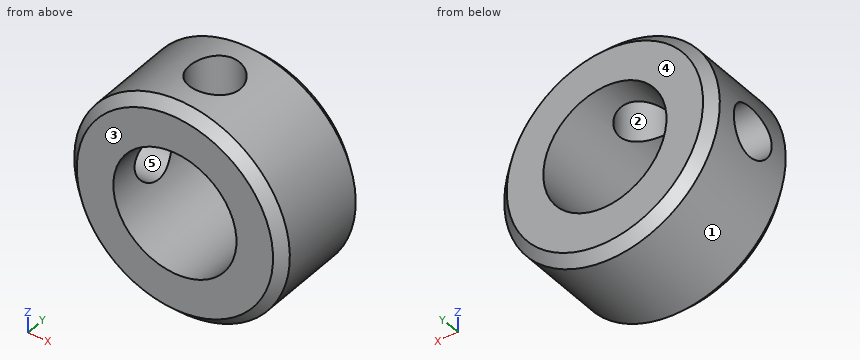
from build123d import *

# Parameters (mm, degrees)
SKETCH1_R                  = 7
SKETCH1_R_2                = 4
BOSS_EXTRUDE1_DEPTH        = 3.5
M4X0_7_TAPPED_HOLE1_REACH  = 18.039
M4X0_7_TAPPED_HOLE1_BORE_R = 1.65
CHAMFER1_SIZE              = 0.625
CIRPATTERN1_COUNT          = 2
CIRPATTERN1_ANGLE          = 90


with BuildPart() as part:
    # Sketch1 → Boss-Extrude1 (new, symmetric)
    with BuildSketch(Plane(origin=(0, 0, 0), x_dir=(1, 0, 0), z_dir=(0, 1, 0))):
        with Locations(Location((0, 0, 0), (0, 0, 270))):
            Circle(SKETCH1_R)
        with Locations(Location((0, 0, 0), (0, 0, 270))):
            Circle(SKETCH1_R_2, mode=Mode.SUBTRACT)
    extrude(amount=BOSS_EXTRUDE1_DEPTH, both=True)

    # M4x0.7 Tapped Hole1 bore → M4x0.7 Tapped Hole1 (cut, up to next)
    with BuildSketch(Plane.XY.offset(7), mode=Mode.PRIVATE) as m4x0_7_tapped_hole1_sk1:
        Circle(M4X0_7_TAPPED_HOLE1_BORE_R)
    m4x0_7_tapped_hole1_tool1 = extrude(m4x0_7_tapped_hole1_sk1.sketch, amount=-M4X0_7_TAPPED_HOLE1_REACH, mode=Mode.PRIVATE) & part.part
    m4x0_7_tapped_hole1 = m4x0_7_tapped_hole1_tool1.solids().sort_by_distance((0, 0, 7))[0]
    add(m4x0_7_tapped_hole1, mode=Mode.SUBTRACT)

    # Chamfer1
    chamfer1_edges = [part.edges().sort_by_distance(p)[0] for p in [
        (0, -3.5, -7),
        (0, 3.5, -7),
    ]]
    chamfer(chamfer1_edges, length=CHAMFER1_SIZE)

    # CirPattern1: M4x0.7 Tapped Hole1 ×2 about axis
    cirpattern1_axis = Axis((0, 3.5, 0), (0, -1, 0))
    for i in range(1, CIRPATTERN1_COUNT):
        add(m4x0_7_tapped_hole1.rotate(cirpattern1_axis, i * CIRPATTERN1_ANGLE / (CIRPATTERN1_COUNT - 1)), mode=Mode.SUBTRACT)


solid = part.part
Build history of the part. All positions in model axes, mm. Face numbers are marked on the shaded views. A direction names the side the tool comes from. Round coordinates to 2 decimals unless told otherwise and drop trailing zeros. Write each loop counter-clockwise with the first axis right and the second up, starting at its lowest first coordinate (ties: lowest second). Pieces come first, ordered by that corner, then holes. Notation, with made-up numbers: M 83.5,0.25 L 108.5,0.25 A26 cw 108.5,26.25 Z; hole C 43,-26 d5. An arc over 180 degrees is marked long. Answer as a JSON object with one key per item and string values. Group by question number.
(1) Cut at B-B (x = 0). Give the cut face in (y, z) (3 decimals).
(2) Which spindle directions (+Z, -Z, +X, -X, +Y, -Y) get a long thin tool onto all of the face, cutting with end or side? Do the marked faces 1 and 2. Say none if no direction does.
(3) Cut at A-A (z = 0). Give the cut face in (x, y) (3 decimals).
(4) Drill centre lines: L1, parallel to Y at x = 0, z = 5.75; L2, parallel to X at y = 1, z = 1.5; L3, parallel to X at y = 2, z = 3. Where is each one in solid material? Low to high.
(5) Flat gauge pins, fed straight in: pin 1 (4 mm diameter, centred on x = 3, y = -2, fed in from -Z); pin 2 (1.5 mm diameter, centred on x = -5, y = 3, fed in from -Z); pin 3 (2 mm diameter, centred on x = 0, y = 0, fed in from +Z). Where does each tip first touch, or does it go through?
(6) Mould opens along Y. For the marked faces 3, 4 and 5 say: pulls with the +Y half, pulls with the -Y half, needs draft (parallel to the pull), parting line crosses it, or undercut.
(7) Cut at C-C (y = -2.25). Give the cut face in (x, z).
Responses:
{
 "1": {"outline": "M -3.5,-6.375 L -2.875,-7 L 2.875,-7 L 3.5,-6.375 L 3.5,-4 L -3.5,-4 Z; M -3.5,4 L -1.65,4 L -1.65,7 L -2.875,7 L -3.5,6.375 Z; M 1.65,4 L 3.5,4 L 3.5,6.375 L 2.875,7 L 1.65,7 Z"},
 "2": {"face 1": "+Y, -Y", "face 2": "+Z"},
 "3": {"outline": "M -7,-2.875 L -6.375,-3.5 L -4,-3.5 L -4,-1.65 L -7,-1.65 Z; M -7,1.65 L -4,1.65 L -4,3.5 L -6.375,3.5 L -7,2.875 Z; M 4,-3.5 L 6.375,-3.5 L 7,-2.875 L 7,2.875 L 6.375,3.5 L 4,3.5 Z"},
 "4": {"L1": "y = -3.5 to -1.65, 1.65 to 3.5", "L2": "x = -6.84 to -3.71, 3.71 to 6.84", "L3": "x = -6.32 to -2.65, 2.65 to 6.32"},
 "5": {"pin 1": "stops at z = -6.93", "pin 2": "stops at z = -5.55", "pin 3": "stops at z = -3.87"},
 "6": {"face 3": "pulls with the -Y half", "face 4": "pulls with the +Y half", "face 5": "undercut"},
 "7": {"outline": "C 0,0 d14; hole C 0,0 d8"}
}
